Input: part model. Units: mm. Frame: model coordinates. Give positions to 0.01 mm unless a question says otherwise; leave off trailing zeros. One line per item, written item: value. Start each with the question number.
(1) Ray query, line 1 along Z through (x, y) = (10.5, 1.2); line 2 along Z through (x, y) = (8, 0.7); line 3 along Z through (x, y) = (11, 0.75). Return the intervals inside material, ascending. Write a range as from..to.
(2) Pin query (flat end, axial travel): P1, Ø4, axis at x = -19.95, z = -19.52, coming from the -Y side; P2, Ø0.8, axis at x = 8.32, z = 22.67, coming from the -Y side. Return the tip coordinate at first contact, or that it passes through.
(3) Section A-A on y = 1.15. State how many separate pieces and enclosed holes the cut face has, plus the area to 3 significant figures.
```python
from build123d import *

# Parameters (mm, degrees)
SKETCH1_W           = 49.657
SKETCH1_H           = 49.403
BOSS_EXTRUDE1_DEPTH = 1.5748
CHAMFER1_SIZE       = 5.08
CHAMFER2_SIZE       = 2.54
SKETCH2_R           = 0.508
CUT_EXTRUDE1_DEPTH  = 36.058501245
SKETCH3_R           = 0.508
SKETCH3_R_2         = 0.4445
CUT_EXTRUDE2_DEPTH  = 2.54


with BuildPart() as part:
    # Sketch1 → Boss-Extrude1 (new body)
    with BuildSketch(Plane(origin=(0, 0, 0), x_dir=(1, 0, 0), z_dir=(0, 1, 0))):
        Rectangle(SKETCH1_W, SKETCH1_H)
    extrude(amount=BOSS_EXTRUDE1_DEPTH)

    # Chamfer1
    chamfer1_edges = [part.edges().sort_by_distance(p)[0] for p in [
        (-24.8285, 0.7874, -24.7015),
        (24.8285, 0.7874, -24.7015),
    ]]
    chamfer(chamfer1_edges, length=CHAMFER1_SIZE)

    # Chamfer2
    chamfer2_edges = [part.edges().sort_by_distance(p)[0] for p in [
        (24.8285, 0.7874, 24.7015),
        (-24.8285, 0.7874, 24.7015),
    ]]
    chamfer(chamfer2_edges, length=CHAMFER2_SIZE)

    # Sketch2 → Cut-Extrude1 (cut, through all)
    with BuildSketch(Plane(origin=(0, 1.5748, 0), x_dir=(1, 0, 0), z_dir=(0, 1, 0))):
        with BuildLine():
            ThreePointArc((-18.4517, 19.5199), (-21.012360172, 20.580560172), (-19.9517, 18.0199))
            Line((-19.9517, 18.0199), (-19.9517, 19.5199))
            Line((-19.9517, 19.5199), (-18.4517, 19.5199))
        make_face()
        with BuildLine():
            Line((-19.9517, 19.5199), (-19.9517, 18.0199))
            ThreePointArc((-19.9517, 18.0199), (-18.891039828, 18.459239828), (-18.4517, 19.5199))
            Line((-18.4517, 19.5199), (-19.9517, 19.5199))
        make_face()
        with BuildLine():
            ThreePointArc((18.6295, 19.5199), (19.068839828, 18.459239828), (20.1295, 18.0199))
            Line((20.1295, 18.0199), (20.1295, 19.5199))
            Line((20.1295, 19.5199), (18.6295, 19.5199))
        make_face()
        with BuildLine():
            Line((20.1295, 19.5199), (20.1295, 18.0199))
            ThreePointArc((20.1295, 18.0199), (21.190160172, 18.459239828), (21.6295, 19.5199))
            ThreePointArc((21.6295, 19.5199), (20.1295, 21.0199), (18.6295, 19.5199))
            Line((18.6295, 19.5199), (20.1295, 19.5199))
        make_face()
        with BuildLine():
            ThreePointArc((20.1295, -19.1883), (19.068839828, -19.627639828), (18.6295, -20.6883))
            Line((18.6295, -20.6883), (20.1295, -20.6883))
            Line((20.1295, -20.6883), (20.1295, -19.1883))
        make_face()
        with BuildLine():
            Line((20.1295, -20.6883), (18.6295, -20.6883))
            ThreePointArc((18.6295, -20.6883), (20.1295, -22.1883), (21.6295, -20.6883))
            ThreePointArc((21.6295, -20.6883), (21.190160172, -19.627639828), (20.1295, -19.1883))
            Line((20.1295, -19.1883), (20.1295, -20.6883))
        make_face()
        with BuildLine():
            Line((-19.9517, -19.1883), (-19.9517, -20.6883))
            Line((-19.9517, -20.6883), (-18.4517, -20.6883))
            ThreePointArc((-18.4517, -20.6883), (-18.891039828, -19.627639828), (-19.9517, -19.1883))
        make_face()
        with BuildLine():
            Line((-18.4517, -20.6883), (-19.9517, -20.6883))
            Line((-19.9517, -20.6883), (-19.9517, -19.1883))
            ThreePointArc((-19.9517, -19.1883), (-21.012360172, -21.748960172), (-18.4517, -20.6883))
        make_face()
        with Locations(Location((5.7785, -20.1295, 0), (0, 0, 270))):
            Circle(SKETCH2_R)
        with Locations(Location((8.3185, -20.1295, 0), (0, 0, 270))):
            Circle(SKETCH2_R)
        with Locations(Location((10.8585, -20.1295, 0), (0, 0, 270))):
            Circle(SKETCH2_R)
        with Locations(Location((13.3985, -20.1295, 0), (0, 0, 270))):
            Circle(SKETCH2_R)
        with Locations(Location((13.3985, -22.6695, 0), (0, 0, 270))):
            Circle(SKETCH2_R)
        with Locations(Location((10.8585, -22.6695, 0), (0, 0, 270))):
            Circle(SKETCH2_R)
        with Locations(Location((8.3185, -22.6695, 0), (0, 0, 270))):
            Circle(SKETCH2_R)
        with Locations(Location((5.7785, -22.6695, 0), (0, 0, 270))):
            Circle(SKETCH2_R)
    extrude(amount=-CUT_EXTRUDE1_DEPTH, mode=Mode.SUBTRACT)

    # Sketch3 → Cut-Extrude2 (cut)
    with BuildSketch(Plane(origin=(0, 1.5748, 0), x_dir=(1, 0, 0), z_dir=(0, 1, 0))):
        with Locations(Location((12.7635, 20.0025, 0), (0, 0, 270))):
            Circle(SKETCH3_R)
        with Locations(Location((7.6835, 20.0025, 0), (0, 0, 270))):
            Circle(SKETCH3_R)
        with Locations(Location((2.6035, 20.0025, 0), (0, 0, 270))):
            Circle(SKETCH3_R)
        with Locations(Location((-2.4765, 20.0025, 0), (0, 0, 270))):
            Circle(SKETCH3_R)
        with Locations(Location((-8.6233, 20.0025, 0), (0, 0, 270))):
            Circle(SKETCH3_R_2)
        with Locations(Location((-13.65137741, 20.0025, 0), (0, 0, 270))):
            Circle(SKETCH3_R_2)
    extrude(amount=-CUT_EXTRUDE2_DEPTH, mode=Mode.SUBTRACT)


solid = part.part
```
Output values:
1. line 1: z = -24.7..19.77, 20.49..22.31, 23.03..24.7
1. line 2: z = -24.7..-20.4, -19.61..19.73, 20.53..22.27, 23.07..24.7
1. line 3: z = -24.7..19.64, 20.62..22.18, 23.16..24.7
2. P1: stops at y = 0
2. P2: passes through
3. separate pieces: 1
3. enclosed holes: 18
3. area: 2,380 mm²
